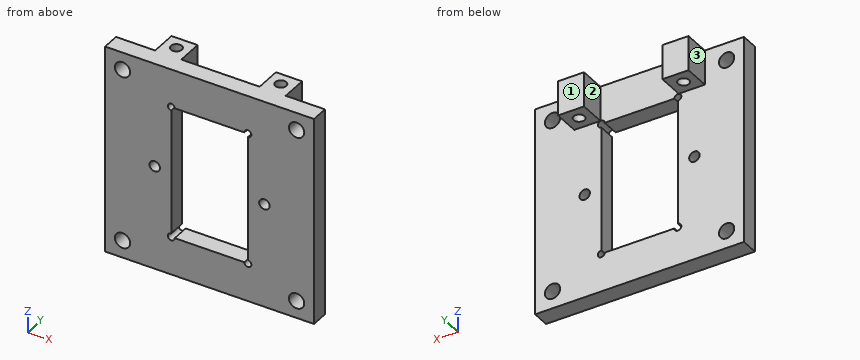
```python
from build123d import *

# Parameters (mm, degrees)
F0_W     = 76.2
F0_H     = 76.2
F3_DEPTH = 6.35
F4_DEPTH = 6.351
F2_R     = 2.794
F5_DEPTH = 6.351
F6_W     = 9.525
F6_H     = 9.525
F6_R     = 2.032
F7_DEPTH = 12.7
F8_R     = 1.905
F9_DEPTH = 6.351


with BuildPart() as f3:
    # F0 (on Front) → F3 (new body)
    with BuildSketch(Plane.XZ):
        Rectangle(F0_W, F0_H)
    extrude(amount=F3_DEPTH)

    # F1 (on Front) → F4 (cut, through all)
    with BuildSketch(Plane.XZ):
        with BuildLine():
            Line((12.7, 24.13), (-12.7, 24.13))
            ThreePointArc((-12.7, 24.13), (-14.868026, 25.028026), (-13.97, 22.86))
            Line((-13.97, 22.86), (-13.97, -22.86))
            ThreePointArc((-13.97, -22.86), (-14.868026, -25.028026), (-12.7, -24.13))
            Line((-12.7, -24.13), (12.7, -24.13))
            ThreePointArc((12.7, -24.13), (14.868026, -25.028026), (13.97, -22.86))
            Line((13.97, -22.86), (13.97, 22.86))
            ThreePointArc((13.97, 22.86), (14.868026, 25.028026), (12.7, 24.13))
        make_face()
    extrude(amount=F4_DEPTH, mode=Mode.SUBTRACT)

    # F2 (on Front) → F5 (cut, through all)
    with BuildSketch(Plane.XZ):
        with Locations((-31.75, 31.75)):
            Circle(F2_R)
        with Locations((-31.75, -31.75)):
            Circle(F2_R)
        with Locations((31.75, -31.75)):
            Circle(F2_R)
        with Locations((31.75, 31.75)):
            Circle(F2_R)
    extrude(amount=F5_DEPTH, mode=Mode.SUBTRACT)

    # F6 (on face) → F7 (join)
    with BuildSketch(Plane.XY.offset(38.1)):
        with Locations((-19.05, 4.7625)):
            Rectangle(F6_W, F6_H)
        with Locations((-19.05, 4.7625)):
            Circle(F6_R, mode=Mode.SUBTRACT)
        with Locations((19.05, 4.7625)):
            Rectangle(F6_W, F6_H)
        with Locations((19.05, 4.7625)):
            Circle(F6_R, mode=Mode.SUBTRACT)
    extrude(amount=-F7_DEPTH)

    # F8 (on Front) → F9 (cut, through all)
    with BuildSketch(Plane.XZ):
        with Locations((-20.0025, 0)):
            Circle(F8_R)
        with Locations((20.0025, 0)):
            Circle(F8_R)
    extrude(amount=F9_DEPTH, mode=Mode.SUBTRACT)


solid = f3.part
```
Work out the finished part from the listing and answer in its coordinate system (mm). Face numbers are marked on the shaded views. Coordinates: 2 decimals unless noted, no trailing zeros. Loops run counter-clockwise (first coordinate to the right, second up) from the corner with the lowest first, then second, coordinate; pieces in that order, holes last. Notation, with made-up numbers: M 81.5,4 L 104.5,4 A14 ccw 104.5,10 Z; hole C 65,54.5 d2. An arc over 180 degrees is marked long. Use CSV: the item, a comma, the result in double quotes. Start each with the question number.
(1) Find section D-D, the plane z = -21. Give the vertices of the cut face in (x, y).
(2) For a pull along X with two mould halves and no side action, classify the marked faces 1, 2 and 3 as +X half, -X half, draft (parallel to the pull), parting line (faces both ways), or undercut.
(3) Find section B-B, the plane z = -31.75. Give the vertices of the cut face in (x, y), then the cut area to 3 significant figures.
(4) Find section A-A, the plane y = 1. Give the vertices of the cut face in (x, z).
(5) Find section C-C, the plane x = -19.05. State how many separate pieces and enclosed holes the cut face has, then the cut area to 3 significant figures.
(6) Given pin 1 Ø3 at (x, z) = (5.5, 27) entering from +Y; pin 2 Ø3 at (x, y) = (-19.5, 4) entering from -Z; pin 3 Ø5 at (y, z) = (5.5, 30.5) entering from +X; pin 4 Ø8 at (x, y) = (19, 0.5) entering from -Z, each flat-ended and moving along its own axis, determine where each tip first touches the part or whether it passes through.
(7) Consider line 1 (X direction, y = -2.5, z = 31.75); line 2 (X direction, y = -2, z = 0). Determine where each line is inside the solid, lowest interval first.
Recorded:
1,outline,"M -38.1,-6.35 L -13.97,-6.35 L -13.97,0 L -38.1,0 Z; M 13.97,-6.35 L 38.1,-6.35 L 38.1,0 L 13.97,0 Z"
2,face 1,"draft"
2,face 2,"undercut"
2,face 3,"-X half"
3,outline,"M -38.1,-6.35 L -34.54,-6.35 L -34.54,0 L -38.1,0 Z; M -28.96,-6.35 L 28.96,-6.35 L 28.96,0 L -28.96,0 Z; M 34.54,-6.35 L 38.1,-6.35 L 38.1,0 L 34.54,0 Z"
3,area,"413 mm^2"
4,outline,"M -23.81,25.4 L -14.29,25.4 L -14.29,38.1 L -23.81,38.1 Z; M 14.29,25.4 L 23.81,25.4 L 23.81,38.1 L 14.29,38.1 Z"
5,separate pieces,"3"
5,enclosed holes,"0"
5,area,"532 mm^2"
6,pin 1,"stops at y = 0"
6,pin 2,"stops at z = 25.4"
6,pin 3,"stops at x = 23.81"
6,pin 4,"stops at z = -38.1"
7,line 1,"x = -38.1 to -34.54, -28.96 to 28.96, 34.54 to 38.1"
7,line 2,"x = -38.1 to -21.91, -18.1 to -13.97, 13.97 to 18.1, 21.91 to 38.1"
